Drawing for the job (mm, zero at the part's lowest x, y, z). A direction names the side the tool comes from. Round coordinates to 2 decimals unless told otherwise and drop trailing zeros. Loops run counter-clockwise (first coordinate to the right, second up) from the corner with the lowest first, then second, coordinate; pieces in that order, holes last. Notation, with made-up numbers: M 4,27.25 L 9,27.25 A20 cw 9,62.25 Z; hole C -34,69 d10. An arc over 180 degrees is marked long. Write each question's results on one line, items separated by ' | '.
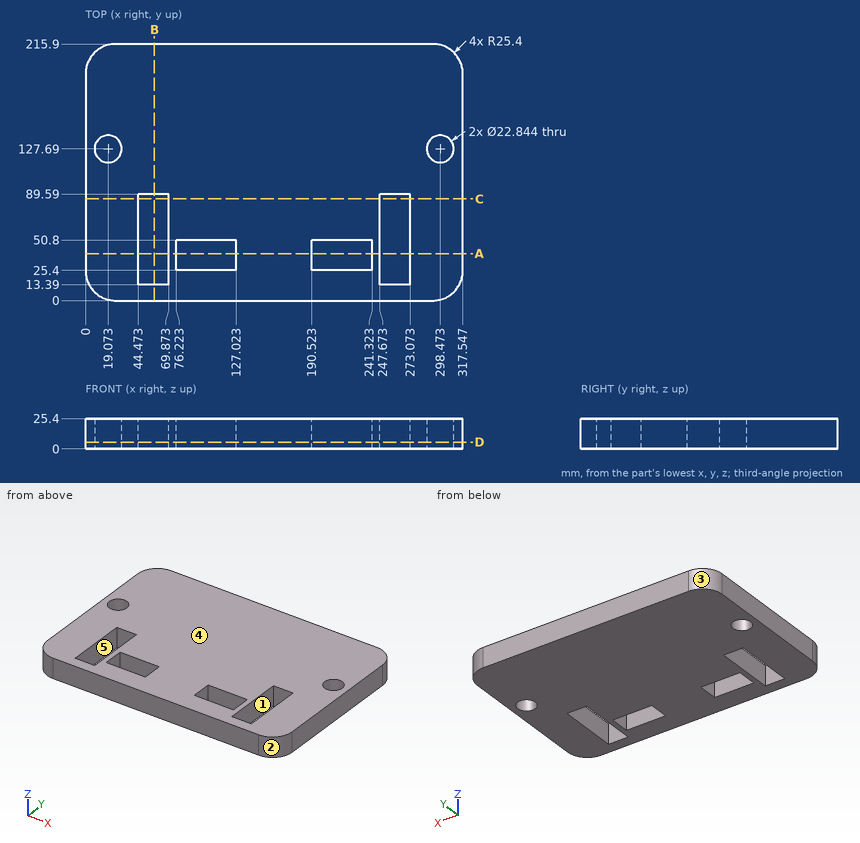
Item 1: Band-saw the part on D-D on z = 5.5. Give the cut face in (x, y) (1 decimal), and give its area (3 significant figures).
Filled sheet:
outline: M 0,25.4 A25.4 ccw 25.4,0 L 292.1,0 A25.4 ccw 317.5,25.4 L 317.5,190.5 A25.4 ccw 292.1,215.9 L 25.4,215.9 A25.4 ccw 0,190.5 Z; hole C 19.1,127.7 d22.8; hole M 44.5,13.4 L 69.9,13.4 L 69.9,89.6 L 44.5,89.6 Z; hole M 76.2,25.4 L 127,25.4 L 127,50.8 L 76.2,50.8 Z; hole M 190.5,25.4 L 241.3,25.4 L 241.3,50.8 L 190.5,50.8 Z; hole M 247.7,13.4 L 273.1,13.4 L 273.1,89.6 L 247.7,89.6 Z; hole C 298.5,127.7 d22.8 | area: 60,700 mm^2
Item 2: Band-saw the part on B-B on x = 58. Give the cut face in (y, z), and give its area (3 significant figures).
Filled sheet:
outline: M 0,0 L 13.39,0 L 13.39,25.4 L 0,25.4 Z; M 89.59,0 L 215.9,0 L 215.9,25.4 L 89.59,25.4 Z | area: 3,550 mm^2
Item 3: Band-saw the part on A-A on y = 39.5. Give the cut face in (x, z).
Filled sheet:
outline: M 0,0 L 44.47,0 L 44.47,25.4 L 0,25.4 Z; M 69.87,0 L 76.22,0 L 76.22,25.4 L 69.87,25.4 Z; M 127.02,0 L 190.52,0 L 190.52,25.4 L 127.02,25.4 Z; M 241.32,0 L 247.67,0 L 247.67,25.4 L 241.32,25.4 Z; M 273.07,0 L 317.55,0 L 317.55,25.4 L 273.07,25.4 Z
Item 4: Wall check: L1, parallel to X at y = 79.5, z = 14; L2, parallel to X at y = 42, z = 7; L3, parallel to Y at x = 53.5, z = 11. Give the ranges that are in metal, low to high.
Filled sheet:
L1: 0 to 44.47, 69.87 to 247.67, 273.07 to 317.55 | L2: 0 to 44.47, 69.87 to 76.22, 127.02 to 190.52, 241.32 to 247.67, 273.07 to 317.55 | L3: 0 to 13.39, 89.59 to 215.9
Item 5: Which spindle directions (+Z, -Z, +X, -X, +Y, -Y) get a long thin tool onto all of the face, cutting with end or side? Do the marked faces 1 and 2. Say none if no direction does.
Filled sheet:
face 1: +Z, -Z | face 2: +Z, -Z, +X, -Y
Item 6: Two-plate mould, pull along Y, no slides. Class the marked faces 3, 4 and 5: +Y half, -Y half, draft (parallel to the pull), parting line (faces both ways), or undercut.
Filled sheet:
face 3: +Y half | face 4: draft | face 5: undercut
Item 7: Band-saw the part on C-C on y = 85.5. Give the cut face in (x, z).
Filled sheet:
outline: M 0,0 L 44.47,0 L 44.47,25.4 L 0,25.4 Z; M 69.87,0 L 247.67,0 L 247.67,25.4 L 69.87,25.4 Z; M 273.07,0 L 317.55,0 L 317.55,25.4 L 273.07,25.4 Z
